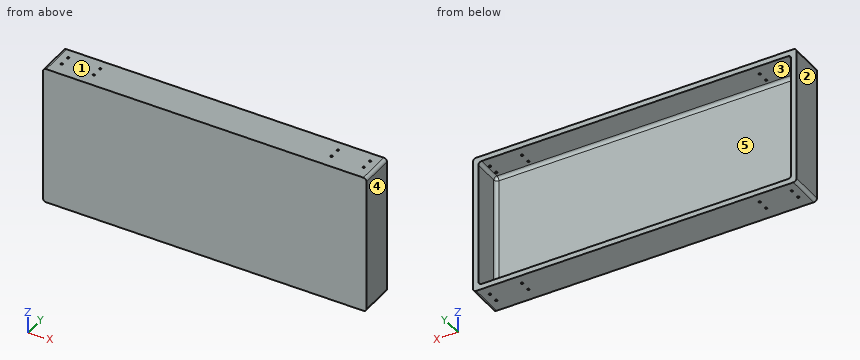
from build123d import *

# Parameters (mm, degrees)
SKETCH1_W           = 300
SKETCH1_H           = 130
BOSS_EXTRUDE1_DEPTH = 32
SHELL1_T            = -5
SKETCH3_R           = 1
CUT_EXTRUDE1_DEPTH  = 202.05720579
FILLET1_R           = 3
FILLET2_R           = 3
FILLET3_R           = 3
FILLET4_R           = 3
FILLET5_R           = 3
FILLET6_R           = 3
FILLET7_R           = 3
FILLET8_R           = 3


with BuildPart() as part:
    # Sketch1 → Boss-Extrude1 (new body)
    with BuildSketch(Plane(origin=(0, 0, 0), x_dir=(1, 0, 0), z_dir=(0, 1, 0))):
        Rectangle(SKETCH1_W, SKETCH1_H)
    extrude(amount=BOSS_EXTRUDE1_DEPTH)

    # Shell1
    shell1_openings = [part.faces().sort_by_distance(p)[0] for p in [
        (0, 32, 0),
    ]]
    offset(amount=SHELL1_T, openings=shell1_openings, kind=Kind.INTERSECTION)

    # Sketch3 → Cut-Extrude1 (cut, through all)
    with BuildSketch(Plane.XY.offset(65)):
        with Locations((-140, 22.4)):
            Circle(SKETCH3_R)
        with Locations((-110.2, 22.4)):
            Circle(SKETCH3_R)
        with Locations((-140, 12.5)):
            Circle(SKETCH3_R)
        with Locations((-110.2, 12.5)):
            Circle(SKETCH3_R)
    cut_extrude1 = extrude(amount=-CUT_EXTRUDE1_DEPTH, mode=Mode.SUBTRACT)

    # Mirror1: Cut-Extrude1 across plane
    add(cut_extrude1.mirror(Plane(origin=(0, 0, 0), x_dir=(0, 0, 1), z_dir=(1, 0, 0))), mode=Mode.SUBTRACT)

    # Fillet1
    fillet1_edges = [part.edges().sort_by_distance(p)[0] for p in [
        (145, 5, 0),
    ]]
    fillet(fillet1_edges, radius=FILLET1_R)

    # Fillet2
    fillet2_edges = [part.edges().sort_by_distance(p)[0] for p in [
        (145, 20, -60),
        (-1.5, 5, -60),
        (144.121320344, 5.878679656, -60),
    ]]
    fillet(fillet2_edges, radius=FILLET2_R)

    # Fillet3
    fillet3_edges = [part.edges().sort_by_distance(p)[0] for p in [
        (-145, 20, -60),
        (-145, 5, 1.5),
        (-145, 5.878679656, -59.121320344),
    ]]
    fillet(fillet3_edges, radius=FILLET3_R)

    # Fillet4
    fillet4_edges = [part.edges().sort_by_distance(p)[0] for p in [
        (0, 5, 60),
        (-144.121320344, 5.878679656, 60),
        (145, 20, 60),
        (-145, 20, 60),
        (144.121320344, 5.878679656, 60),
    ]]
    fillet(fillet4_edges, radius=FILLET4_R)

    # Fillet5
    fillet5_edges = [part.edges().sort_by_distance(p)[0] for p in [
        (150, 16, -65),
    ]]
    fillet(fillet5_edges, radius=FILLET5_R)

    # Fillet6
    fillet6_edges = [part.edges().sort_by_distance(p)[0] for p in [
        (-150, 16, -65),
    ]]
    fillet(fillet6_edges, radius=FILLET6_R)

    # Fillet7
    fillet7_edges = [part.edges().sort_by_distance(p)[0] for p in [
        (-150, 16, 65),
    ]]
    fillet(fillet7_edges, radius=FILLET7_R)

    # Fillet8
    fillet8_edges = [part.edges().sort_by_distance(p)[0] for p in [
        (150, 16, 65),
    ]]
    fillet(fillet8_edges, radius=FILLET8_R)


solid = part.part
CAD build for the part. Positions are in the model's coordinates, mm. Face numbers are marked on the shaded views. A direction names the side the tool comes from. Coordinates: 2 decimals unless noted, no trailing zeros. Write each loop counter-clockwise with the first axis right and the second up, starting at its lowest first coordinate (ties: lowest second). Pieces come first, ordered by that corner, then holes. Notation, with made-up numbers: (0.5, -8.5) - (37.5, -8.5) arc R13 cw to (37.5, 13.5) - close; hole circle Ø1 at (-32.75, 64). An arc over 180 degrees is marked (long way). Use a Markdown table: item, result. Add a question column.
Item 1: Drill centre lines: L1, parallel to Y at x = -110.2, z = 62; L2, parallel to Z at x = -133.5, y = 22.5; L3, parallel to X at y = 18.5, z = 31.5. Where is each one in solid material? Low to high. Write a range as from..to.
Item 2: Band-saw the part on B-B, the plane x = -59.5. Give the cut face in (y, z).
Item 3: Band-saw the part on A-A, the plane z = 4.5. Give the cut face in (x, y).
Item 4: Mould opens along X. For the marked faces 1, 2 and 3 say: pulls with the +X half, pulls with the -X half, needs draft (parallel to the pull), parting line crosses it, or undercut.
Item 5: 3-axis set-ups, long thin cutter, end or side, ignore diameter. For the marked faces 4 and 5: which of +Z, -Z, +X, -X, +Y, -Y reach the whole face in a straight line?
Item 6: Flat gauge pin, fed straight in: pin 1 (10 mm diameter, centred on x = -29, z = -30.5, fed in from +Y). Where does the tip first touch, or does it go through?
Numbers:
| question | item | result |
|---|---|---|
| 1 | L1 | 0..11.5, 13.5..21.4, 23.4..32 |
| 1 | L2 | -65..-60, 60..65 |
| 1 | L3 | -150..-145, 145..150 |
| 2 | outline | (0, -65) - (32, -65) - (32, -60) - (8, -60) arc R3 cw to (5, -57) - (5, 57) arc R3 cw to (8, 60) - (32, 60) - (32, 65) - (0, 65) - close |
| 3 | outline | (-150, 0) - (150, 0) - (150, 32) - (145, 32) - (145, 8) arc R3 cw to (142, 5) - (-142, 5) arc R3 cw to (-145, 8) - (-145, 32) - (-150, 32) - close |
| 4 | face 1 | needs draft |
| 4 | face 2 | pulls with the -X half |
| 4 | face 3 | undercut |
| 5 | face 4 | +Z, -Z, +X, +Y, -Y |
| 5 | face 5 | +Y |
| 6 | pin 1 | y = 5 |
